Here's the drawing with two shaded views (mm, measured from the low corner). I have some questions. A direction names the side the tool comes from. Coordinates: 2 decimals unless noted, no trailing zeros. Write each loop counter-clockwise with the first axis right and the second up, starting at its lowest first coordinate (ties: lowest second). Pieces come first, ordered by that corner, then holes. Notation, with made-up numbers: (46.25, 4) -> (69.25, 4) arc R38 cw to (69.25, 42) -> close; hole circle Ø10 at (11, 42.25). An arc over 180 degrees is marked (long way). Use one line per item in the form item = value.
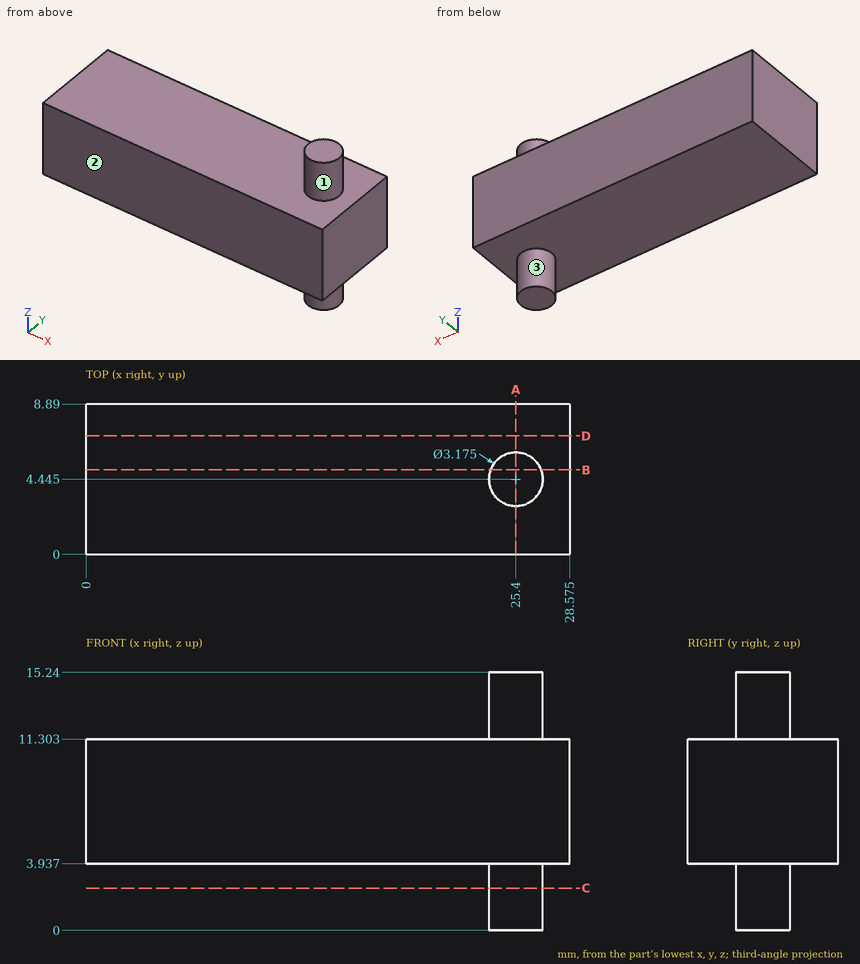
Q1. Will these pins go through, and if not, where does the flat tip stop? pin 1 (3 mm diameter, centred on x = 13, y = 7.5, fed in from +Z); pin 2 (1 mm diameter, centred on y = 1.5, z = 2, fed in from -X); pin 3 (2 mm diameter, centred on x = 4, y = 5.5, fed in from -Z).
Return value:
pin_1 = 11.3
pin_2 = through
pin_3 = 3.94
Q2. Suppose I cut it at D-D (y = 7). Write out the boundary of the cut face in (x, z) (3 decimals), then the cut area to 3 significant figures.
Return value:
outline = (0, 3.937) -> (28.575, 3.937) -> (28.575, 11.303) -> (0, 11.303) -> close
area = 210 mm2
Q3. Suppose I cut it at B-B (y = 5). Write out the boundary of the cut face in (x, z) (3 decimals).
Return value:
outline = (0, 3.937) -> (23.913, 3.937) -> (23.913, 0) -> (26.887, 0) -> (26.887, 3.937) -> (28.575, 3.937) -> (28.575, 11.303) -> (26.887, 11.303) -> (26.887, 15.24) -> (23.913, 15.24) -> (23.913, 11.303) -> (0, 11.303) -> close
Q4. Suppose I cut it at A-A (x = 25.4). Write out the boundary of the cut face in (y, z).
Return value:
outline = (0, 3.94) -> (2.86, 3.94) -> (2.86, 0) -> (6.03, 0) -> (6.03, 3.94) -> (8.89, 3.94) -> (8.89, 11.3) -> (6.03, 11.3) -> (6.03, 15.24) -> (2.86, 15.24) -> (2.86, 11.3) -> (0, 11.3) -> close
Q5. Suppose I cut it at C-C (z = 2.5). Write out the boundary of the cut face in (x, y) (1 decimal).
Return value:
outline = circle Ø3.2 at (25.4, 4.4)
Q6. If I drill on line 1 (Z direction, x = 22.5, y = 3); line 2 (X direction, y = 3.5, z = 13.25); line 3 (Y direction, x = 24, z = 14.5), over which ranges is the centre line in solid material (lowest first)? Write a range as from..to.
Return value:
line_1 = 3.94..11.3
line_2 = 24.12..26.68
line_3 = 3.7..5.19
Q7. For the marked faces 1, 2 and 3, which set-ups out of +Z, -Z, +X, -X, +Y, -Y let a thin tool reach every point of the face, with its end or its side?
Return value:
face_1 = +Z
face_2 = +Z, -Z, +X, -X, -Y
face_3 = -Z
